Work out the finished part from the listing and answer in its coordinate system (mm). Give positions to 0.01 mm unless a question says otherwise; leave off trailing zeros. Loops run counter-clockwise (first coordinate to the right, second up) from the corner with the lowest first, then second, coordinate; pieces in that order, holes last. Notation, with made-up numbers: M 26.25,54.25 L 31.25,54.25 A22 cw 31.25,85.25 Z; hole C 21.5,48.25 d2. An arc over 180 degrees is marked long. Write item = value, one per line. Start each with the question number.
1. The mould has two halves that part along X. Classify faces 1 (the face through (52.31, 9.04, 2.54)), 2 (the face through (30, 37, 2)), 3 (the face through (60, 18, 2)): released by +X, released by -X, zero draft, split by the parting line, or undercut.
2. Section A-A on z = 2.7 is taken. Determine the outline of the cut face in (x, y).
3. Section B-B on y = 32.5 is taken. Determine the outline of the cut face in (x, z), plus the area to 3 significant figures.
4. Flat-ended cylindrical pins translate along their axes: pin 1 Ø1.5 at (x, z) = (6.5, 2) entering from -Y; pin 2 Ø2 at (x, y) = (43.5, 8.5) entering from -Z. Find the tip coordinate at first contact, or state that the pin passes through.
5. Consider L1, parallel to Y at x = 50, z = 3.95; L2, parallel to X at y = 11.5, z = 2.9; L3, parallel to X at y = 5, z = 1.85. Determine where each line is inside the solid, lowest interval first. Write a range as [from, to].
Autodesk Inventor part; units mm, degrees
ref_plane "YZ Plane" through (0, 0, 0) normal (1, 0, 0) x (0, 1, 0)
ref_plane "XZ Plane" through (0, 0, 0) normal (0, 1, 0) x (-1, 0, 0)
ref_plane "XY Plane" through (0, 0, 0) normal (0, 0, 1) x (1, 0, 0)
sketch "Sketch1" plane through (0, 0, 0) normal (0, 0, 1) x (1, 0, 0)
  line L0 (0, 0) -> (60, 0)
  line L1 (60, 0) -> (60, 37)
  line L2 (60, 37) -> (0, 37)
  line L3 (0, 37) -> (0, 0)
  dimension "d0" = 60
  dimension "d1" = 37
extrude "Extrusion1" add sketch "Sketch1" along normal blind 5
sketch "Sketch2" plane through (0, 0, 5) normal (0, 0, 1) x (1, 0, 0)
  circle A0 centre (10, 10) radius 2.5
  circle A1 centre (50, 10) radius 2.5
  circle A2 centre (10, 27) radius 2.5
  circle A3 centre (50, 27) radius 2.5
  point P0 (0, 0)
  dimension "d4" = 5
  dimension "d5" = 5
  dimension "d6" = 5
  dimension "d7" = 5
extrude "Extrusion2" cut sketch "Sketch2" against normal blind 5
fillet "Fillet1" radius 10 1 edges at (0, 37, 2.5)
fillet "Fillet2" radius 10 1 edges at (60, 37, 2.5)
fillet "Fillet3" radius 10 1 edges at (60, 0, 2.5)
fillet "Fillet4" radius 10 1 edges at (0, 0, 2.5)
properties part number "sail_hold_2"
Verdict:
q1.face_1 = undercut
q1.face_2 = zero draft
q1.face_3 = released by +X
q2.outline = M 0,10 A10 ccw 10,0 L 50,0 A10 ccw 60,10 L 60,27 A10 ccw 50,37 L 10,37 A10 ccw 0,27 Z; hole C 10,10 d5; hole C 10,27 d5; hole C 50,10 d5; hole C 50,27 d5
q3.outline = M 1.65,0 L 58.35,0 L 58.35,5 L 1.65,5 Z
q3.area = 284 mm2
q4.pin_1 = 0.39
q4.pin_2 = 0
q5.L1 = [0, 7.5], [12.5, 24.5], [29.5, 37]
q5.L2 = [0, 8], [12, 48], [52, 60]
q5.L3 = [1.34, 58.66]
